Geometry check sheet. Reference: drawing and pictorial views, mm from the part's lowest x, y, z. A direction names the side the tool comes from. Give positions to 0.01 mm unless a question says otherwise; leave off trailing zeros. Loops run counter-clockwise (first coordinate to the right, second up) from the corner with the lowest first, then second, coordinate; pieces in that order, holes last. Notation, with made-up numbers: (25, 87.25) - (44, 87.25) arc R26 ccw to (44, 105.25) - close; hole circle Ø10 at (7, -19). An arc over 180 degrees is marked (long way). One line per question, with ' | ' between items. Start each with the question number.
1. Depth check by flat-ended pin: pin 1 Ø10 at (x, z) = (23.5, 44.5) entering from +Y; pin 2 Ø10 at (y, z) = (25.5, 45.5) entering from -X; pin 3 Ø6 at (y, z) = (33.5, 13) entering from -X. Enter the tip coordinate at first touch or a pass-through.
2. Tool access check on the marked faces 4, 5 and 6. Record the directions out of +Z, -Z, +X, -X, +Y, -Y that give a thin tool (end or side, any length) a straight path to the whole face; none if there is none.
3. Section check A-A, the plane z = 32. Enter the section's corners in (x, y).
4. Section check D-D, the plane x = 32. State how many separate pieces and enclosed holes the cut face has, then the cut area to 3 significant figures.
5. Section check B-B, the plane x = 19.5. Enter the section's corners in (y, z).
6. Thickness scan on line 1 along Z through (x, y) = (32, 8.75); line 2 along Z through (x, y) = (49.5, 9.5); line 3 along Y through (x, z) = (32, 13.5). Record the ranges inside material, lowest first. Write a range as from..to.
7. Section check C-C, the plane y = 23. Enter the section's corners in (x, z), then the cut area to 3 significant figures.
8. Mould release check, pull along Z, two halves, no side actions. Record for the marked faces 1, 2 and 3: +Z half, -Z half, draft (parallel to the pull), parting line (faces both ways), or undercut.
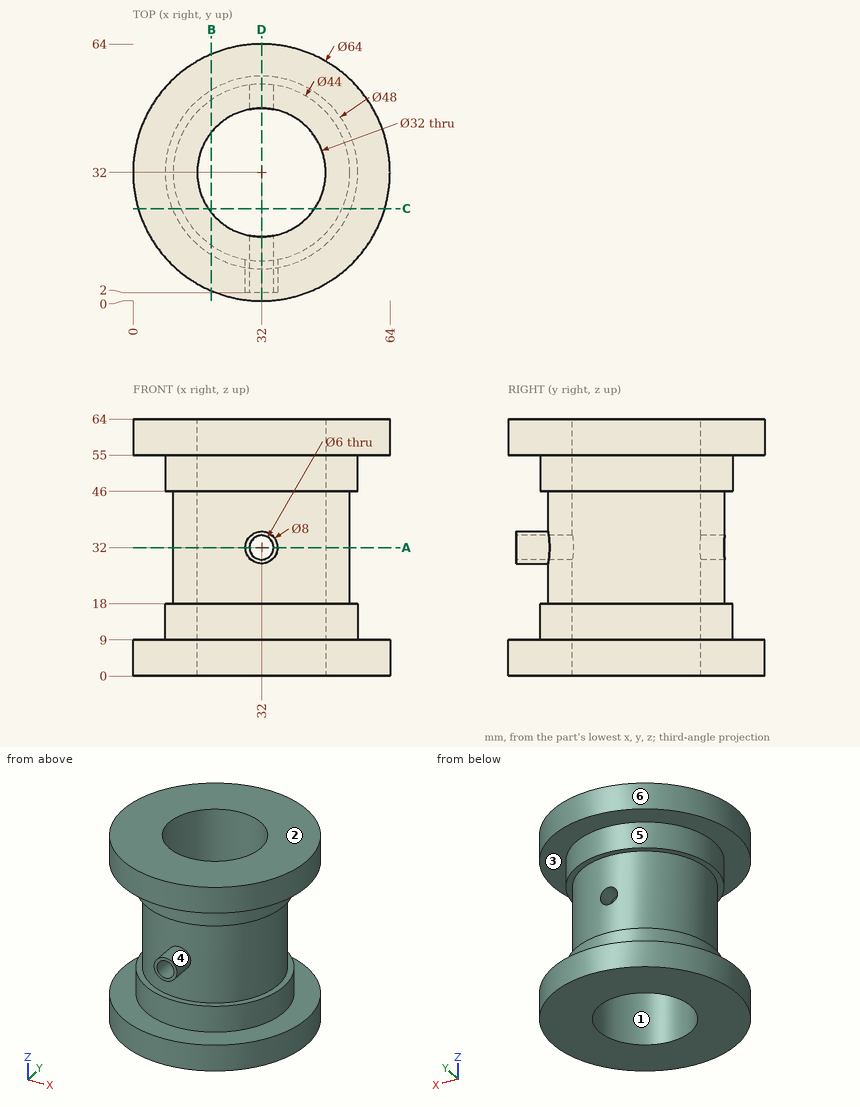
Results list:
1) pin 1: y = 55.71 | pin 2: x = 8.05 | pin 3: x = 8
2) face 4: -Y | face 5: none | face 6: +Z, -Z
3) outline: (28, 2) - (29, 2) - (29, 16.28) arc R16 cw to (29, 47.72) - (29, 53.79) arc R22 ccw to (28, 10.37) - close; (35, 2) - (36, 2) - (36, 10.37) arc R22 ccw to (35, 53.79) - (35, 47.72) arc R16 cw to (35, 16.28) - close
4) separate pieces: 4 | enclosed holes: 0 | area: 1,140 mm²
5) outline: (2.54, 0) - (22.01, 0) - (22.01, 64) - (2.54, 64) - (2.54, 55) - (11.51, 55) - (11.51, 46) - (13.9, 46) - (13.9, 18) - (11.51, 18) - (11.51, 9) - (2.54, 9) - close; (41.99, 0) - (61.46, 0) - (61.46, 9) - (52.49, 9) - (52.49, 18) - (50.1, 18) - (50.1, 46) - (52.49, 46) - (52.49, 55) - (61.46, 55) - (61.46, 64) - (41.99, 64) - close
6) line 1: 0..18, 28..29, 35..36, 46..64 | line 2: 0..9, 55..64 | line 3: 8..16, 48..56
7) outline: (1.29, 0) - (18.77, 0) - (18.77, 64) - (1.29, 64) - (1.29, 55) - (9.75, 55) - (9.75, 46) - (11.93, 46) - (11.93, 18) - (9.75, 18) - (9.75, 9) - (1.29, 9) - close; (45.23, 0) - (62.71, 0) - (62.71, 9) - (54.25, 9) - (54.25, 18) - (52.07, 18) - (52.07, 46) - (54.25, 46) - (54.25, 55) - (62.71, 55) - (62.71, 64) - (45.23, 64) - close | area: 1,340 mm²
8) face 1: draft | face 2: +Z half | face 3: undercut
